```python
from build123d import *

# Parameters (mm, degrees)
SKETCH1_R           = 3
BOSS_EXTRUDE1_DEPTH = 10


with BuildPart() as part:
    # Sketch1 → Boss-Extrude1 (new body)
    with BuildSketch(Plane.XY):
        with BuildLine():
            Line((0, 14.498076211), (1.186155793, 12.443594112))
            ThreePointArc((1.186155793, 12.443594112), (1.188200541, 12.443399032), (1.190245258, 12.443203616))
            Line((1.190245258, 12.443203616), (2.743778964, 14.236077087))
            Line((2.743778964, 14.236077087), (3.519686083, 11.994240696))
            ThreePointArc((3.519686083, 11.994240696), (3.521656961, 11.99366217), (3.523627743, 11.99308332))
            Line((3.523627743, 11.99308332), (5.388390607, 13.459549045))
            Line((5.388390607, 13.459549045), (5.726005747, 11.111384171))
            ThreePointArc((5.726005747, 11.111384171), (5.727831522, 11.110443108), (5.729657142, 11.109501746))
            Line((5.729657142, 11.109501746), (7.838251774, 12.196557832))
            Line((7.838251774, 12.196557832), (7.725372644, 9.826933271))
            ThreePointArc((7.725372644, 9.826933271), (7.726987328, 9.825663684), (7.728601803, 9.824393833))
            Line((7.728601803, 9.824393833), (10.0048181, 10.492751241))
            Line((10.0048181, 10.492751241), (9.445524446, 8.187311399))
            ThreePointArc((9.445524446, 8.187311399), (9.446869679, 8.185759174), (9.448214658, 8.184206729))
            Line((9.448214658, 8.184206729), (11.809784233, 8.409709282))
            Line((11.809784233, 8.409709282), (10.824290385, 6.251778761))
            ThreePointArc((10.824290385, 6.251778761), (10.825317547, 6.25), (10.826344418, 6.248221071))
            Line((10.826344418, 6.248221071), (13.187913993, 6.022718518))
            Line((13.187913993, 6.022718518), (11.811838266, 4.090290549))
            ThreePointArc((11.811838266, 4.090290549), (11.812510234, 4.088349541), (11.813181883, 4.086408423))
            Line((11.813181883, 4.086408423), (14.089398181, 3.418051015))
            Line((14.089398181, 3.418051015), (12.372475537, 1.780968581))
            ThreePointArc((12.372475537, 1.780968581), (12.372768024, 1.778935478), (12.373060176, 1.776902328))
            Line((12.373060176, 1.776902328), (14.481654809, 0.689846242))
            Line((14.481654809, 0.689846242), (12.485939306, -0.592722233))
            ThreePointArc((12.485939306, -0.592722233), (12.48584174, -0.594773948), (12.485743836, -0.596825646))
            Line((12.485743836, -0.596825646), (14.3505067, -2.063291371))
            Line((14.3505067, -2.063291371), (12.148128697, -2.944990521))
            ThreePointArc((12.148128697, -2.944990521), (12.147644604, -2.946986694), (12.147160183, -2.948982787))
            Line((12.147160183, -2.948982787), (13.70069389, -4.741856258))
            Line((13.70069389, -4.741856258), (11.371253065, -5.190819178))
            ThreePointArc((11.371253065, -5.190819178), (11.370399942, -5.192687663), (11.369546512, -5.194556007))
            Line((11.369546512, -5.194556007), (12.555702305, -7.249038106))
            Line((12.555702305, -7.249038106), (10.183390719, -7.249038106))
            ThreePointArc((10.183390719, -7.249038106), (10.182199401, -7.25071137), (10.181007807, -7.252384438))
            Line((10.181007807, -7.252384438), (10.956914926, -9.494220829))
            Line((10.956914926, -9.494220829), (8.627474101, -9.045257909))
            ThreePointArc((8.627474101, -9.045257909), (8.625987644, -9.046675476), (8.624500953, -9.048092799))
            Line((8.624500953, -9.048092799), (8.962116093, -11.396257674))
            Line((8.962116093, -11.396257674), (6.75973809, -10.514558524))
            ThreePointArc((6.75973809, -10.514558524), (6.758010218, -10.51566916), (6.756282164, -10.516779513))
            Line((6.756282164, -10.516779513), (6.643403034, -12.886404074))
            Line((6.643403034, -12.886404074), (4.647687532, -11.603835599))
            ThreePointArc((4.647687532, -11.603835599), (4.645780696, -11.604599163), (4.643873734, -11.605362413))
            Line((4.643873734, -11.605362413), (4.08458008, -13.910802256))
            Line((4.08458008, -13.910802256), (2.367657437, -12.273719822))
            ThreePointArc((2.367657437, -12.273719822), (2.365640555, -12.274108716), (2.363623608, -12.274497278))
            Line((2.363623608, -12.274497278), (1.37812976, -14.4324278))
            Line((1.37812976, -14.4324278), (0.002054033, -12.499999831))
            ThreePointArc((0.002054033, -12.499999831), (0, -12.5), (-0.002054033, -12.499999831))
            Line((-0.002054033, -12.499999831), (-1.37812976, -14.4324278))
            Line((-1.37812976, -14.4324278), (-2.363623608, -12.274497278))
            ThreePointArc((-2.363623608, -12.274497278), (-2.365640555, -12.274108716), (-2.367657437, -12.273719822))
            Line((-2.367657437, -12.273719822), (-4.08458008, -13.910802256))
            Line((-4.08458008, -13.910802256), (-4.643873734, -11.605362413))
            ThreePointArc((-4.643873734, -11.605362413), (-4.645780696, -11.604599163), (-4.647687532, -11.603835599))
            Line((-4.647687532, -11.603835599), (-6.643403034, -12.886404074))
            Line((-6.643403034, -12.886404074), (-6.756282164, -10.516779513))
            ThreePointArc((-6.756282164, -10.516779513), (-6.758010218, -10.51566916), (-6.75973809, -10.514558524))
            Line((-6.75973809, -10.514558524), (-8.962116093, -11.396257674))
            Line((-8.962116093, -11.396257674), (-8.624500953, -9.048092799))
            ThreePointArc((-8.624500953, -9.048092799), (-8.625987644, -9.046675476), (-8.627474101, -9.045257909))
            Line((-8.627474101, -9.045257909), (-10.956914926, -9.494220829))
            Line((-10.956914926, -9.494220829), (-10.181007807, -7.252384438))
            ThreePointArc((-10.181007807, -7.252384438), (-10.182199401, -7.25071137), (-10.183390719, -7.249038106))
            Line((-10.183390719, -7.249038106), (-12.555702305, -7.249038106))
            Line((-12.555702305, -7.249038106), (-11.369546512, -5.194556007))
            ThreePointArc((-11.369546512, -5.194556007), (-11.370399942, -5.192687663), (-11.371253065, -5.190819178))
            Line((-11.371253065, -5.190819178), (-13.70069389, -4.741856258))
            Line((-13.70069389, -4.741856258), (-12.147160183, -2.948982787))
            ThreePointArc((-12.147160183, -2.948982787), (-12.147644604, -2.946986694), (-12.148128697, -2.944990521))
            Line((-12.148128697, -2.944990521), (-14.3505067, -2.063291371))
            Line((-14.3505067, -2.063291371), (-12.485743836, -0.596825646))
            ThreePointArc((-12.485743836, -0.596825646), (-12.48584174, -0.594773948), (-12.485939306, -0.592722233))
            Line((-12.485939306, -0.592722233), (-14.481654809, 0.689846242))
            Line((-14.481654809, 0.689846242), (-12.373060176, 1.776902328))
            ThreePointArc((-12.373060176, 1.776902328), (-12.372768024, 1.778935478), (-12.372475537, 1.780968581))
            Line((-12.372475537, 1.780968581), (-14.089398181, 3.418051015))
            Line((-14.089398181, 3.418051015), (-11.813181883, 4.086408423))
            ThreePointArc((-11.813181883, 4.086408423), (-11.812510234, 4.088349541), (-11.811838266, 4.090290549))
            Line((-11.811838266, 4.090290549), (-13.187913993, 6.022718518))
            Line((-13.187913993, 6.022718518), (-10.826344418, 6.248221071))
            ThreePointArc((-10.826344418, 6.248221071), (-10.825317547, 6.25), (-10.824290385, 6.251778761))
            Line((-10.824290385, 6.251778761), (-11.809784233, 8.409709282))
            Line((-11.809784233, 8.409709282), (-9.448214658, 8.184206729))
            ThreePointArc((-9.448214658, 8.184206729), (-9.446869679, 8.185759174), (-9.445524446, 8.187311399))
            Line((-9.445524446, 8.187311399), (-10.0048181, 10.492751241))
            Line((-10.0048181, 10.492751241), (-7.728601803, 9.824393833))
            ThreePointArc((-7.728601803, 9.824393833), (-7.726987328, 9.825663684), (-7.725372644, 9.826933271))
            Line((-7.725372644, 9.826933271), (-7.838251774, 12.196557832))
            Line((-7.838251774, 12.196557832), (-5.729657142, 11.109501746))
            ThreePointArc((-5.729657142, 11.109501746), (-5.727831522, 11.110443108), (-5.726005747, 11.111384171))
            Line((-5.726005747, 11.111384171), (-5.388390607, 13.459549045))
            Line((-5.388390607, 13.459549045), (-3.523627743, 11.99308332))
            ThreePointArc((-3.523627743, 11.99308332), (-3.521656961, 11.99366217), (-3.519686083, 11.994240696))
            Line((-3.519686083, 11.994240696), (-2.743778964, 14.236077087))
            Line((-2.743778964, 14.236077087), (-1.190245258, 12.443203616))
            ThreePointArc((-1.190245258, 12.443203616), (-1.188200541, 12.443399032), (-1.186155793, 12.443594112))
            Line((-1.186155793, 12.443594112), (0, 14.498076211))
        make_face()
        Circle(SKETCH1_R, mode=Mode.SUBTRACT)
    extrude(amount=BOSS_EXTRUDE1_DEPTH)


solid = part.part
```
The model under review builds one solid part; all positions refer to its coordinate system, in mm. A direction names the side the tool comes from. Round coordinates to 2 decimals unless told otherwise and drop trailing zeros. Loops run counter-clockwise (first coordinate to the right, second up) from the corner with the lowest first, then second, coordinate; pieces in that order, holes last. Notation, with made-up numbers: (52.5, -39.5) -> (108.5, -39.5) arc R15 ccw to (108.5, -23.5) -> close; hole circle Ø10 at (8, 17). An arc over 180 degrees is marked (long way). Answer as a JSON object with one key per item and string values. Group by question number.
1) For faces 4 (the face through (12.51, 5.07, 4.93)), 5 (the face through (-0.68, -13.45, 4.93)), 6 (the face through (0.58, 13.49, 4.93)), 7 (the face through (-11.31, 7.32, 4.93)), list the 3-axis set-ups (+Z, -Z, +X, -X, +Y, -Y) from which the entire face can be reached by the end or side of a thin tool; tool diameter is ignored.
2) Mouldability with a two-part tool opening along Y and no side actions: class faces 1 (the face through (-6.8, 11.66, 4.93)), 2 (the face through (5.66, -12.254, 4.93)), 3 (the face through (12.935, 3.757, 4.93)) as released by +Y, released by -Y, zero draft, split by the parting line, or undercut.
3) For line 1 (Y direction, x = 13, z = 8.5); line 2 (Y direction, x = 0.75, z = 1.75); line 3 (X direction, y = -12.75, z = 4.5), list the stretches that pass through material, from the lowest coordinate up. Write a range as [from, to].
4) We need section A-A on y = 0. Write out the cut boundary in (x, z), then the cut area to 3 significant figures.
5) For pin 1 Ø0.7 at (x, z) = (-12, 6) entering from -Y; pin 2 Ø2 at (y, z) = (3, 7) entering from -X; pin 3 Ø2.5 at (x, z) = (11.5, 7) entering from -Y, all flat-tipped, find the tip position at first contact; note any pin that passes through.
6) We need section B-B on x = -0.75. Write out the cut boundary in (y, z), then the cut area to 3 significant figures.
Result set:
{
 "1": {"face 4": "+Z, -Z, +X", "face 5": "+Z, -Z, -Y", "face 6": "+Z, -Z, +Y", "face 7": "+Z, -Z, -X"},
 "2": {"face 1": "released by +Y", "face 2": "released by -Y", "face 3": "undercut"},
 "3": {"line 1": "[-4.88, -3.93], [-2.6, -1], [-0.26, 1.45], [2.38, 3.74], [5.76, 6.04]", "line 2": "[-13.55, -2.9], [2.9, 13.2]", "line 3": "[-6.65, -6.43], [-4.37, -2.87], [-2.15, -0.18], [0.18, 2.15], [2.87, 4.37], [6.43, 6.65]"},
 "4": {"outline": "(-13.41, 0) -> (-3, 0) -> (-3, 10) -> (-13.41, 10) -> close; (3, 0) -> (13.41, 0) -> (13.41, 10) -> (3, 10) -> close", "area": "208 mm²"},
 "5": {"pin 1": "y = -7.25", "pin 2": "x = -14.09", "pin 3": "y = -9.49"},
 "6": {"outline": "(-13.55, 0) -> (-2.9, 0) -> (-2.9, 10) -> (-13.55, 10) -> close; (2.9, 0) -> (13.2, 0) -> (13.2, 10) -> (2.9, 10) -> close", "area": "209 mm²"}
}
